The listing builds one solid part. Answer for the finished solid, in the listing's coordinates (mm). A direction names the side the tool comes from. Give positions to 0.01 mm unless a question says otherwise; leave off trailing zeros. Order: outer loops, then holes, each group sorted by start corner. A loop starts at its lowest first (then second) coordinate and runs counter-clockwise, first axis right, second up. Notation, with made-up numbers: (-33.5, 53) - (19.5, 53) arc R24 ccw to (19.5, 68) - close; hole circle Ø7 at (-36.75, -33). An arc over 180 degrees is marked (long way). Write each question's results on one line, items separated by ' | '. Start each with the question number.
1. Flat-ended cylindrical pins translate along their axes: pin 1 (4.5 mm diameter, centred on x = 33.5, y = -15, fed in from -Z); pin 2 (1.2 mm diameter, centred on x = 33.7, y = -15.7, fed in from +Z); pin 3 (6 mm diameter, centred on x = 18, y = -7.5, fed in from +Z). Find the tip coordinate at first contact, or state that the pin passes through.
2. Which of the six approach directions +Z, -Z, +X, -X, +Y, -Y give full straight-line access (tool end or side, diameter ignored) to faces 4 (the face through (-32.14, -14.1, -16.48)), 5 (the face through (-33.917, 14.724, -15.986)), 6 (the face through (35.547, -14.934, -18.521))?
3. Find the intervals of material crossed by L1, parallel to Y at x = 33.7, z = -15.9; L2, parallel to Y at x = -33.7, z = -17.65; L3, parallel to X at y = 15.7, z = -18.35, in increasing order.
4. Determine the mould class of faces 1 (the face through (1, 0, -20)), 2 (the face through (-32.777, 17.474, -18.521)), 3 (the face through (-35.248, 17.287, -17.535)) for opening direction X: released by +X, released by -X, zero draft, split by the parting line, or undercut.
5. Section D-D (z = -16.1) is taken. Give the vertices of the cut face in (x, y), and give its area (3 significant figures).
6. Section A-A (z = -19.05) is taken. Give the vertices of the cut face in (x, y), and give its area (3 significant figures).
7. Section B-B (x = -16) is taken. Give the vertices of the cut face in (y, z), and give its area (3 significant figures).
8. Section C-C (y = -7) is taken. Give the vertices of the cut face in (x, z).
from build123d import *

# Parameters (mm, degrees)
PAD002_DEPTH    = 5
SKETCH012_R     = 1
POCKET008_DEPTH = 20.001
SKETCH013_R     = 2
POCKET009_DEPTH = 3
POCKET010_DEPTH = 3


with BuildPart() as part:
    # Sketch010 → Pad002 (new body)
    with BuildSketch(Plane.XY.offset(-20)):
        with BuildLine():
            Line((-33.5, 18), (33.5, 18))
            ThreePointArc((36, 15.5), (35.267767, 17.267767), (33.5, 18))
            Line((36, 15.5), (36, -15.5))
            ThreePointArc((33.5, -18), (35.267767, -17.267767), (36, -15.5))
            Line((33.5, -18), (-33.5, -18))
            ThreePointArc((-36, -15.5), (-35.267767, -17.267767), (-33.5, -18))
            Line((-36, -15.5), (-36, 15.5))
            ThreePointArc((-33.5, 18), (-35.267767, 17.267767), (-36, 15.5))
        make_face()
    extrude(amount=PAD002_DEPTH)

    # Sketch012 (on Pad) → Pocket008 (cut, through all)
    with BuildSketch(Plane.XY):
        with Locations((-33.7, 15.7)):
            Circle(SKETCH012_R)
        with Locations((33.7, 15.7)):
            Circle(SKETCH012_R)
        with Locations((33.7, -15.7)):
            Circle(SKETCH012_R)
        with Locations((-33.7, -15.7)):
            Circle(SKETCH012_R)
    extrude(amount=-POCKET008_DEPTH, mode=Mode.SUBTRACT)

    # Sketch013 (on Face4 of Pocket008) → Pocket009 (cut)
    with BuildSketch(Plane(origin=(0, 0, -20), x_dir=(1, 0, 0), z_dir=(0, 0, -1))):
        with Locations((-33.7, 15.7)):
            Circle(SKETCH013_R)
        with Locations((33.7, 15.7)):
            Circle(SKETCH013_R)
        with Locations((33.7, -15.7)):
            Circle(SKETCH013_R)
        with Locations((-33.7, -15.7)):
            Circle(SKETCH013_R)
    extrude(amount=-POCKET009_DEPTH, mode=Mode.SUBTRACT)

    # Sketch011 (on Face10 of Pad002) → Pocket010 (cut)
    with BuildSketch(Plane.XY.offset(-15)):
        with BuildLine():
            Line((33, 12), (33, -12))
            ThreePointArc((30, -15), (32.12132, -14.12132), (33, -12))
            Line((30, -15), (-30, -15))
            ThreePointArc((-33, -12), (-32.12132, -14.12132), (-30, -15))
            Line((-33, -10.5), (-33, -12))
            ThreePointArc((-33, -10.5), (-29.5, -7), (-33, -3.5))
            Line((-33, 12), (-33, -3.5))
            ThreePointArc((-30, 15), (-32.125281, 14.125281), (-33, 12))
            Line((-30, 15), (-25, 15))
            Line((-25, 15), (-25, 9))
            Line((-25, 9), (-12, 9))
            Line((-12, 9), (-12, 15))
            Line((-12, 15), (30, 15))
            ThreePointArc((33, 12), (32.12132, 14.12132), (30, 15))
        make_face()
    extrude(amount=-POCKET010_DEPTH, mode=Mode.SUBTRACT)


solid = part.part
Reported:
1) pin 1: z = -20 | pin 2: through | pin 3: z = -18
2) face 4: +Z | face 5: +Z, -Z | face 6: -Z
3) L1: -17.99 to -16.7, -14.7 to 14.7, 16.7 to 17.99 | L2: -17.99 to -17.7, -13.7 to 13.7, 17.7 to 17.99 | L3: -35.99 to -35.7, -31.7 to 31.7, 35.7 to 35.99
4) face 1: zero draft | face 2: undercut | face 3: released by -X
5) outline: (-36, -15.5) arc R2.5 ccw to (-33.5, -18) - (33.5, -18) arc R2.5 ccw to (36, -15.5) - (36, 15.5) arc R2.5 ccw to (33.5, 18) - (-33.5, 18) arc R2.5 ccw to (-36, 15.5) - close; hole circle Ø2 at (-33.7, -15.7); hole circle Ø2 at (-33.7, 15.7); hole (-33, -12) arc R3 ccw to (-30, -15) - (30, -15) arc R3 ccw to (33, -12) - (33, 12) arc R3 ccw to (30, 15) - (-12, 15) - (-12, 9) - (-25, 9) - (-25, 15) - (-30, 15) arc R2.99 ccw to (-33, 12) - (-33, -3.5) arc R3.5 cw to (-33, -10.5) - close; hole circle Ø2 at (33.7, -15.7); hole circle Ø2 at (33.7, 15.7) | area: 699 mm²
6) outline: (-36, -15.5) arc R2.5 ccw to (-33.5, -18) - (33.5, -18) arc R2.5 ccw to (36, -15.5) - (36, 15.5) arc R2.5 ccw to (33.5, 18) - (-33.5, 18) arc R2.5 ccw to (-36, 15.5) - close; hole circle Ø4 at (-33.7, -15.7); hole circle Ø4 at (-33.7, 15.7); hole circle Ø4 at (33.7, -15.7); hole circle Ø4 at (33.7, 15.7) | area: 2,540 mm²
7) outline: (-18, -20) - (18, -20) - (18, -15) - (9, -15) - (9, -18) - (-15, -18) - (-15, -15) - (-18, -15) - close | area: 108 mm²
8) outline: (-36, -20) - (36, -20) - (36, -15) - (33, -15) - (33, -18) - (-29.5, -18) - (-29.5, -15) - (-36, -15) - close
